For this review, take the finished solid that the model builds, in its own axes (mm). A direction names the side the tool comes from. Coordinates: 2 decimals unless noted, no trailing zeros. Order: outer loops, then holes, each group sorted by start corner. A loop starts at its lowest first (then second) coordinate and runs counter-clockwise, first axis right, second up. Notation, with made-up numbers: M -30,47.25 L -21,47.25 A13 ccw -21,68.25 Z; hole C 7.25,81.25 d10. An arc over 180 degrees is marked long. Use one line per item in the form item = value. Start each with the question number.
```python
from build123d import *
from build123d.topology import SkipClean

# Parameters (mm, degrees)
EXTRUDE_2_DEPTH      = 40
EXTRUDE_2_DEPTH_BACK = 40
SKETCH_1_W           = 150
SKETCH_1_H           = 10
EXTRUDE_3_DEPTH      = 14
EXTRUDE_4_DEPTH      = 14
SKETCH_4_W           = 2
SKETCH_4_H           = 52
EXTRUDE_5_DEPTH      = 24
SKETCH_5_R           = 22
CUT_EXTRUDE_1_DEPTH  = 81
CUT_EXTRUDE_6_DEPTH  = 8
SKETCH_7_W           = 69
SKETCH_7_H           = 55
SKETCH_7_W_2         = 65.5
SKETCH_7_H_2         = 52
EXTRUDE_6_DEPTH      = 4
SKETCH_12_W          = 66
SKETCH_12_H          = 1.5
EXTRUDE_8_DEPTH      = 5
CUT_EXTRUDE_7_DEPTH  = 6
CUT_EXTRUDE_START    = -6
CUT_EXTRUDE_8_DEPTH  = 6
SKETCH_15_R          = 1.1
CUT_EXTRUDE_9_DEPTH  = 4
SKETCH_16_W          = 15.246183725
SKETCH_16_H          = 18.547486822
CUT_EXTRUDE_10_DEPTH = 2
SKETCH_17_W          = 13.790442518
SKETCH_17_H          = 12.65745234
CUT_EXTRUDE_11_DEPTH = 8
EXTRUDE_9_DEPTH      = 24


with BuildPart() as part:
    # Sketch 1 → Extrude 2 (new, two sides: drawn at the far end of the back side and taken through both)
    with BuildSketch(Plane(origin=(0, 0, 0), x_dir=(0, 0, -1), z_dir=(1, 0, 0)).offset(-EXTRUDE_2_DEPTH_BACK)):
        with Locations((0, 29)):
            Rectangle(SKETCH_1_W, SKETCH_1_H)
    extrude(amount=EXTRUDE_2_DEPTH + EXTRUDE_2_DEPTH_BACK)

    # Sketch 3 → Extrude 4 (add)
    with BuildSketch(Plane.ZY.offset(40)):
        with BuildLine():
            Line((-26, 0), (-22, 0))
            ThreePointArc((-22, 0), (0, 22), (22, 0))
            Line((22, 0), (26, 0))
            ThreePointArc((26, 0), (0, 26), (-26, 0))
        make_face()
    extrude(amount=-EXTRUDE_4_DEPTH)



with BuildPart() as body_2:
    # Sketch 2 → Extrude 3 (new body)
    with BuildSketch(Plane(origin=(40, 0, 0), x_dir=(0, 0, -1), z_dir=(1, 0, 0))):
        with BuildLine():
            Line((-26, 0), (-22, 0))
            ThreePointArc((-22, 0), (0, 22), (22, 0))
            Line((22, 0), (26, 0))
            ThreePointArc((26, 0), (0, 26), (-26, 0))
        make_face()
    extrude(amount=-EXTRUDE_3_DEPTH)


with BuildPart() as part_1:
    add(part.part)

    add(body_2.part)  # Extrude 5 merges body 2
    # Sketch 4 → Extrude 5 (add)
    with BuildSketch(Plane(origin=(0, 24, 0), x_dir=(-1, 0, 0), z_dir=(0, -1, 0))):
        with Locations((39, 0)):
            Rectangle(SKETCH_4_W, SKETCH_4_H)
        with Locations((-39, 0)):
            Rectangle(SKETCH_4_W, SKETCH_4_H)
    extrude(amount=EXTRUDE_5_DEPTH)

    # Sketch 5 → Cut-Extrude 1 (cut)
    with SkipClean():  # the faces are left unmerged after this step: merging them gives an invalid solid
        with BuildSketch(Plane(origin=(40, 0, 0), x_dir=(0, 0, -1), z_dir=(1, 0, 0))):
            Circle(SKETCH_5_R)
        extrude(amount=-CUT_EXTRUDE_1_DEPTH, mode=Mode.SUBTRACT)
    add(part_1.part.scale(1), mode=Mode.REPLACE)  # the faces are merged on a copy

    # Sketch 6 → Cut-Extrude 6 (cut)
    with BuildSketch(Plane(origin=(0, 24, 0), x_dir=(-1, 0, 0), z_dir=(0, -1, 0))):
        Polygon((38, 28), (36, 28), (36, 13), (24, 13), (24, -13), (36, -13), (36, -28), (38, -28), (38, -73), (-38, -73), (-38, -27.999124699), (-36, -27.999124699), (-36, -13), (-24, -13), (-24, 13), (-36, 13), (-36, 28), (-38, 28), (-38, 73), (38, 73), align=None)
    extrude(amount=-CUT_EXTRUDE_6_DEPTH, mode=Mode.SUBTRACT)

    # Sketch 7 → Extrude 6 (add)
    with BuildSketch(Plane.XZ.offset(-32)):
        with Locations((5.5, 39)):
            Rectangle(SKETCH_7_W, SKETCH_7_H)
        with Locations((5.25, 39)):
            Rectangle(SKETCH_7_W_2, SKETCH_7_H_2, mode=Mode.SUBTRACT)
    extrude(amount=EXTRUDE_6_DEPTH)

    # Sketch 12 → Extrude 8 (add)
    with BuildSketch(Plane.XY.offset(13)):
        with Locations((5, 28.788266855)):
            Rectangle(SKETCH_12_W, SKETCH_12_H)
    extrude(amount=EXTRUDE_8_DEPTH)

    # Sketch 13 → Cut-Extrude 7 (cut)
    with BuildSketch(Plane(origin=(40, 0, 0), x_dir=(0, 0, -1), z_dir=(1, 0, 0))):
        with BuildLine():
            Line((-24, 0), (-22, 0))
            ThreePointArc((-22, 0), (0, 22), (22, 0))
            Line((22, 0), (24, 0))
            ThreePointArc((24, 0), (0, 24), (-24, 0))
        make_face()
    extrude(amount=-CUT_EXTRUDE_7_DEPTH, mode=Mode.SUBTRACT)

    # Sketch 14 → Cut-Extrude 8 (cut)
    with BuildSketch(Plane.ZY.offset(40).offset(CUT_EXTRUDE_START)):
        with BuildLine():
            Line((-24, 0), (-22, 0))
            ThreePointArc((-22, 0), (0, 22), (22, 0))
            Line((22, 0), (24, 0))
            ThreePointArc((24, 0), (0, 24), (-24, 0))
        make_face()
    extrude(amount=CUT_EXTRUDE_8_DEPTH, mode=Mode.SUBTRACT)

    # Sketch 15 → Cut-Extrude 9 (cut)
    with BuildSketch(Plane.XZ.offset(-32)):
        with Locations(Location((-24, 61.5, 0), (0, 0, 270))):
            Circle(SKETCH_15_R)
    extrude(amount=-CUT_EXTRUDE_9_DEPTH, mode=Mode.SUBTRACT)

    # Sketch 16 → Cut-Extrude 10 (cut)
    with BuildSketch(Plane.XZ.offset(-32)):
        with Locations((30.376908138, 22.273743411)):
            Rectangle(SKETCH_16_W, SKETCH_16_H)
    extrude(amount=CUT_EXTRUDE_10_DEPTH, mode=Mode.SUBTRACT)

    # Sketch 17 → Cut-Extrude 11 (cut)
    with BuildSketch(Plane.XZ.offset(-24)):
        with Locations((31.104778741, 24.32872617)):
            Rectangle(SKETCH_17_W, SKETCH_17_H)
    extrude(amount=-CUT_EXTRUDE_11_DEPTH, mode=Mode.SUBTRACT)

    # Sketch 18 → Extrude 9 (add)
    with BuildSketch(Plane.XZ.offset(-24)):
        Polygon((-40, -24), (-38, -24), (-38, -26), (-38, -73), (38, -73), (38, -26), (38, -24), (40, -24), (40, -75), (-40, -75), align=None)
        Polygon((-40, 75), (40, 75), (40, 26), (40, 24), (38, 24), (38, 26), (38, 73), (-38, 73), (-38, 26), (-38, 24), (-40, 24), (-40, 26), align=None)
    extrude(amount=EXTRUDE_9_DEPTH)


solid = part_1.part
```
1. The part is to be moulded in two halves that separate along Y. For faces 4 (the flat face through (1, 17, -75)), 5 (the flat face through (0, 0, 74)), 6 (the flat face through (-36, 28, 20)), say which applies: pulls with the +Y half, pulls with the -Y half, needs draft (parallel to the pull), parting line crosses it, or undercut.
2. To check wall thickness, follow line 1 (X direction, y = 32.5, z = 61.5); line 2 (Z direction, x = 32.5, y = 29.5); line 3 (X direction, y = 31, z = -55). State the ranges of each line that lie inside material, in increasing order.
3. Tool access review of faces 1 (the flat face through (-30, 28, -13)), 2 (the flat face through (5, 30, 65)), 3 (the flat face through (0, 0, -74)): name each direction out of +Z, -Z, +X, -X, +Y, -Y from which nothing blocks a thin tool from reaching the whole face with its end or side.
4. Consider section B-B, the plane y = 25.5. Write out the cut boundary in (x, z), plus the area to 3 significant figures.
5. For pin 1 Ø19 at (y, z) = (12, -3) entering from -X; pin 2 Ø4 at (x, z) = (-30.5, 8.5) entering from -Y; pin 3 Ø15.5 at (x, z) = (28, -12.5) entering from -Y; pin 4 Ø5 at (x, z) = (-20, -8.5) entering from -Y, all flat-tipped, find the tip position at first contact; note any pin that passes through.
6. Consider section A-A, the plane z = 0. Write out the cut boundary in (x, y).
Answers follow:
q1.face_4 = needs draft
q1.face_5 = pulls with the -Y half
q1.face_6 = undercut
q2.line_1 = -40 to -25.1, -22.9 to 40
q2.line_2 = -75 to -73, -13 to 18, 65 to 66.5, 73 to 75
q2.line_3 = -40 to -38, 38 to 40
q3.face_1 = none
q3.face_2 = -Y
q3.face_3 = +Z, -Z, +X, -X, -Y
q4.outline = M -40,-75 L 40,-75 L 40,75 L -40,75 Z; hole M -38,-73 L 38,-73 L 38,-28 L 36,-28 L 36,-13 L 24,-13 L 24,13 L 36,13 L 36,18 L 38,18 L 38,73 L -38,73 L -38,28 L -36,28 L -36,13 L -24,13 L -24,-13 L -36,-13 L -36,-28 L -38,-28 Z
q4.area = 1,730 mm²
q5.pin_1 = through
q5.pin_2 = 19.33
q5.pin_3 = 8.6
q5.pin_4 = 32
q6.outline = M -40,24 L -34,24 L -34,22 L -26,22 L -26,24 L -24,24 L -24,32 L 24,32 L 24,24 L 26,24 L 26,22 L 34,22 L 34,24 L 40,24 L 40,34 L -40,34 Z
